```python
from build123d import *

# Parameters (mm, degrees)
SKETCH_R           = 8.5
PAD_DEPTH          = 2
SKETCH001_R        = 2
PAD001_DEPTH       = 3
SKETCH002_R        = 9.5
PAD002_DEPTH       = 3.5
PAD003_DEPTH       = 5.5
POLARPATTERN_COUNT = 21
SKETCH005_R        = 9.5
PAD004_DEPTH       = 3
SKETCH006_R        = 1.5
POCKET_DEPTH       = 14.001


with BuildPart() as part:
    # Sketch → Pad (new body)
    with BuildSketch(Plane.XY):
        Circle(SKETCH_R)
    extrude(amount=PAD_DEPTH)

    # Sketch001 → Pad001 (new body)
    with BuildSketch(Plane(origin=(0, 0, 0), x_dir=(1, 0, 0), z_dir=(0, 0, -1))):
        with Locations((0, 6)):
            Circle(SKETCH001_R)
        with Locations((6, 0)):
            Circle(SKETCH001_R)
        with Locations((0, -6)):
            Circle(SKETCH001_R)
        with Locations((-6, 0)):
            Circle(SKETCH001_R)
    extrude(amount=PAD001_DEPTH)

    # Sketch002 → Pad002 (new body)
    with BuildSketch(Plane.XY.offset(2)):
        Circle(SKETCH002_R)
    extrude(amount=PAD002_DEPTH)

    # Sketch004 → Pad003 (new body)
    with BuildSketch(Plane.XY.offset(5.5)):
        with BuildLine():
            ThreePointArc((2.252349, 7.321374), (1.731707, 8.178679), (0.90828, 7.60596))
            ThreePointArc((0.90828, 7.60596), (0.454943, 7.646478), (0, 7.66))
            Line((0, 7.66), (0, 0))
            Line((0, 0), (2.252349, 7.321374))
        make_face()
    pad003 = extrude(amount=PAD003_DEPTH)

    # PolarPattern: Pad003 ×21 about axis
    polarpattern_axis = Axis((0, 0, 5.5), (0, 0, 1))
    for i in range(1, POLARPATTERN_COUNT):
        add(pad003.rotate(polarpattern_axis, i * 360 / POLARPATTERN_COUNT))

    # Sketch005 → Pad004 (new body)
    with BuildSketch(Plane.XY.offset(11)):
        Circle(SKETCH005_R)
    extrude(amount=PAD004_DEPTH)

    # Sketch006 → Pocket (cut, through all)
    with BuildSketch(Plane(origin=(0, 0, 0), x_dir=(1, 0, 0), z_dir=(0, 0, -1))):
        Circle(SKETCH006_R)
    extrude(amount=-POCKET_DEPTH, mode=Mode.SUBTRACT)


solid = part.part
```
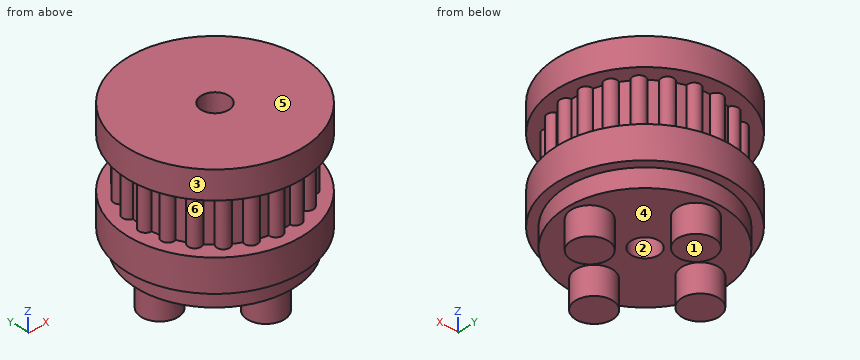
Check sheet for the modelled part. Datum: model origin and axes. Units: mm. Face numbers are marked on the shaded views. A direction names the side the tool comes from. Round coordinates to 2 decimals unless told otherwise and drop trailing zeros. Loops run counter-clockwise (first coordinate to the right, second up) from the corner with the lowest first, then second, coordinate; pieces in that order, holes last. Notation, with made-up numbers: (-38, 78) - (12, 78) arc R8 cw to (12, 86) - close; hole circle Ø4 at (7, -3.5). An arc over 180 degrees is marked (long way). Answer as a JSON object with one key per item and string values. Group by question number.
Q1. Mould release check, pull along Y, two halves, no side actions. Record for the marked faces 1, 2 and 3: released by +Y, released by -Y, zero draft, split by the parting line, or undercut.
Q2. Gauge pin test, flat ends, axial feed: P1, Ø10, axis at x = 6.5, z = 2, coming from the +Y side; P2, Ø4, axis at x = 5.5, y = 5.5, coming from the -Z side; P3, Ø2.5, axis at x = 0, y = 0, coming from the +Z side; P4, Ø1.5, axis at y = -1, z = 2, coming from the -X side. Record the tip position at first contact, or that the pin passes through.
Q3. Sectioned sample at B-B, the plane z = 8.5. Count the separate pieces of the cut face and the enclosed holes in it, plus the area to 3 significant figures.
Q4. Set-up check for the marked faces 4, 5 and 6: record each of +Z, -Z, +X, -X, +Y, -Y from which the full face is reachable in a straight line by a thin tool's end or side.
Q5. Scan lines: line 1 along Z through (x, y) = (-8.5, 1); line 2 along Y through (x, z) = (0, 4); line 3 along Z through (x, y) = (-5.5, 5.5). Record each from-to range of solid material in increasing order. Write a range as [from, to].
Q6. Sectioned sample at A-A, the plane z = 3. Enter the section's corners in (x, y).
Solution:
{
 "1": {"face 1": "zero draft", "face 2": "undercut", "face 3": "split by the parting line"},
 "2": {"P1": "stops at y = 9.38", "P2": "stops at z = 0", "P3": "passes through", "P4": "stops at x = -9.5"},
 "3": {"separate pieces": "21", "enclosed holes": "0", "area": "193 mm²"},
 "4": {"face 4": "-Z", "face 5": "+Z, +X, -X, +Y, -Y", "face 6": "none"},
 "5": {"line 1": "z = [2, 5.5], [11, 14]", "line 2": "y = [-9.5, -1.5], [1.5, 9.5]", "line 3": "z = [0, 5.5], [11, 14]"},
 "6": {"outline": "circle Ø19 at (0, 0); hole circle Ø3 at (0, 0)"}
}
